```python
from build123d import *

# Parameters (mm, degrees)
F0_W     = 50
F0_H     = 60
F1_DEPTH = 12.5
F3_DEPTH = 12.5
F5_DEPTH = 60


# Not quite as in the source:
# - a feature names something its author has since deleted; it is built from what else it names


with BuildPart() as f1:
    # F0 (on Front) → F1 (new body, symmetric)
    with BuildSketch(Plane.XZ):
        with Locations((25, 30)):
            Rectangle(F0_W, F0_H)
    extrude(amount=F1_DEPTH, both=True)

    # F2 (on Right) → F3 (cut, symmetric)
    with BuildSketch(Plane.YZ):
        Polygon((-12.1228452772, 60.4202598333), (0, 60.6142282486), (0, 70.6142282486), align=None)
    extrude(amount=F3_DEPTH, both=True, mode=Mode.SUBTRACT)

    # F4 (on Top) → F5 (cut, through all)
    with BuildSketch(Plane.XY):
        with BuildLine():
            ThreePointArc((30, -2.5), (28.232233047, -6.767766953), (32.5, -5))
            ThreePointArc((32.5, -5), (31.767766953, -3.232233047), (30, -2.5))
        make_face()
    extrude(amount=F5_DEPTH, mode=Mode.SUBTRACT)


solid = f1.part
```
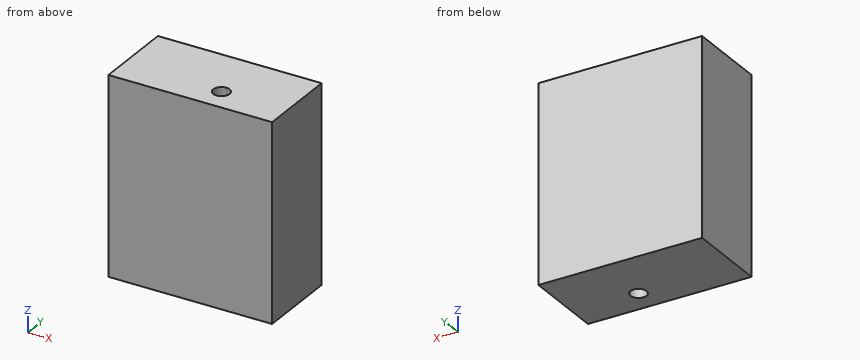
Check sheet for the modelled part. Datum: model origin and axes. Units: mm. Give positions to 0.01 mm unless a question says otherwise; leave off trailing zeros. Write each loop counter-clockwise with the first axis right and the second up, starting at its lowest first coordinate (ties: lowest second). Pieces come first, ordered by that corner, then holes.
Item 1: Cross-section at B-B (y = -3.75). Enter the section's corners in (x, z), and give its area (3 significant figures).
Item 2: Scan lines: L1, parallel to X at y = -5, z = 42; L2, parallel to Y at x = 30, z = 22; L3, parallel to X at y = -6.5, z = 57.5. Record each from-to range of solid material in increasing order.
Item 3: Cross-section at A-A (z = 49.5). Enter the section's corners in (x, y), and give its area (3 significant figures).
Report:
1. outline: (0, 0) - (27.83, 0) - (27.83, 60) - (0, 60) - close; (32.17, 0) - (50, 0) - (50, 60) - (32.17, 60) - close
1. area: 2,740 mm2
2. L1: x = 0 to 27.5, 32.5 to 50
2. L2: y = -12.5 to -7.5, -2.5 to 12.5
2. L3: x = 0 to 28, 32 to 50
3. outline: (0, -12.5) - (50, -12.5) - (50, 12.5) - (0, 12.5) - close; hole circle Ø5 at (30, -5)
3. area: 1,230 mm2
